Source: CAD feature listing. Evaluate the final solid. Frame: model axes, mm. Face numbers are marked on the shaded views. Give positions to 0.01 mm unless a question says otherwise; leave off trailing zeros. Order: outer loops, then holes, each group sorted by start corner. A loop starts at its lowest first (then second) coordinate and runs counter-clockwise, first axis right, second up.
from build123d import *

# Parameters (mm, degrees)
SALIENTE_EXTRUIR1_DEPTH = 75
SALIENTE_EXTRUIR2_START = -17
SALIENTE_EXTRUIR2_DEPTH = 17.566243
CROQUIS3_R              = 3.96875
CORTAR_EXTRUIR1_DEPTH   = 10
CROQUIS4_R              = 6.46875
CROQUIS4_R_2            = 3.96875
CORTAR_EXTRUIR2_DEPTH   = 3
SALIENTE_EXTRUIR3_START = -6.919182
CROQUIS7_R              = 1.984375
SALIENTE_EXTRUIR3_DEPTH = 6.919182
CORTAR_EXTRUIR3_DEPTH   = 75
CROQUIS9_R              = 1
CORTAR_EXTRUIR4_DEPTH   = 10


with BuildPart() as part:
    # Croquis1 → Saliente-Extruir1 (new body, symmetric)
    with BuildSketch(Plane.XY):
        with BuildLine():
            ThreePointArc((-1.339746, 5), (14.365661, 8.57646), (28, 0))
            Line((28, 0), (28, -10))
            Line((28, -10), (25, -10))
            Line((25, -10), (25, 0))
            Line((25, 0), (0, 0))
            Line((0, 0), (-60.621778, -35))
            Line((-60.621778, -35), (-70.621778, -35))
            Line((-70.621778, -35), (-1.339746, 5))
        make_face()
    extrude(amount=SALIENTE_EXTRUIR1_DEPTH, both=True)

    # Croquis2 → Saliente-Extruir2 (add)
    with BuildSketch(Plane(origin=(0, -15, 0), x_dir=(1, 0, 0), z_dir=(0, 1, 0)).offset(SALIENTE_EXTRUIR2_START)):
        with BuildLine():
            Line((-32.5, 4.330127), (-32.5, 12.5))
            Line((-32.5, 12.5), (-27.5, 12.5))
            Line((-27.5, 12.5), (-27.5, 4.330127))
            ThreePointArc((-27.5, 4.330127), (-25, 0), (-27.5, -4.330127))
            Line((-27.5, -4.330127), (-27.5, -12.5))
            Line((-27.5, -12.5), (-32.5, -12.5))
            Line((-32.5, -12.5), (-32.5, -4.330127))
            ThreePointArc((-32.5, -4.330127), (-35, 0), (-32.5, 4.330127))
        make_face()
        with BuildLine():
            Line((-32.5, 54.330127), (-32.5, 62.5))
            Line((-32.5, 62.5), (-27.5, 62.5))
            Line((-27.5, 62.5), (-27.5, 54.330127))
            ThreePointArc((-27.5, 54.330127), (-25, 50), (-27.5, 45.669873))
            Line((-27.5, 45.669873), (-27.5, 37.5))
            Line((-27.5, 37.5), (-32.5, 37.5))
            Line((-32.5, 37.5), (-32.5, 45.669873))
            ThreePointArc((-32.5, 45.669873), (-35, 50), (-32.5, 54.330127))
        make_face()
        with BuildLine():
            Line((-32.5, -45.669873), (-32.5, -37.5))
            Line((-32.5, -37.5), (-27.5, -37.5))
            Line((-27.5, -37.5), (-27.5, -45.669873))
            ThreePointArc((-27.5, -45.669873), (-25, -50), (-27.5, -54.330127))
            Line((-27.5, -54.330127), (-27.5, -62.5))
            Line((-27.5, -62.5), (-32.5, -62.5))
            Line((-32.5, -62.5), (-32.5, -54.330127))
            ThreePointArc((-32.5, -54.330127), (-35, -50), (-32.5, -45.669873))
        make_face()
    extrude(amount=SALIENTE_EXTRUIR2_DEPTH)

    # Croquis3 → Cortar-Extruir1 (cut)
    with BuildSketch(Plane(origin=(0, 8.875562, 0), x_dir=(1, 0, 0), z_dir=(0, 1, 0))):
        with Locations((14, -50)):
            Circle(CROQUIS3_R)
        with Locations((14, 0)):
            Circle(CROQUIS3_R)
        with Locations((14, 50)):
            Circle(CROQUIS3_R)
    extrude(amount=-CORTAR_EXTRUIR1_DEPTH, mode=Mode.SUBTRACT)

    # Croquis4 → Cortar-Extruir2 (cut)
    with BuildSketch(Plane(origin=(0, 8.875562, 0), x_dir=(1, 0, 0), z_dir=(0, 1, 0))):
        with Locations((14, 50)):
            Circle(CROQUIS4_R)
        with Locations((14, 50)):
            Circle(CROQUIS4_R_2, mode=Mode.SUBTRACT)
        with Locations((14, 0)):
            Circle(CROQUIS4_R)
        with Locations((14, 0)):
            Circle(CROQUIS4_R_2, mode=Mode.SUBTRACT)
        with Locations((14, -50)):
            Circle(CROQUIS4_R)
        with Locations((14, -50)):
            Circle(CROQUIS4_R_2, mode=Mode.SUBTRACT)
    extrude(amount=-CORTAR_EXTRUIR2_DEPTH, mode=Mode.SUBTRACT)

    # Croquis7 → Saliente-Extruir3 (add)
    with BuildSketch(Plane(origin=(0, -35, 0), x_dir=(-1, 0, 0), z_dir=(0, -1, 0)).offset(SALIENTE_EXTRUIR3_START)):
        with Locations((50.621778, 0)):
            Circle(CROQUIS7_R)
        with Locations((50.621778, 50)):
            Circle(CROQUIS7_R)
        with Locations((50.621778, -50)):
            Circle(CROQUIS7_R)
    extrude(amount=SALIENTE_EXTRUIR3_DEPTH)

    # Croquis8 → Cortar-Extruir3 (cut, symmetric)
    with BuildSketch(Plane.XY):
        with BuildLine():
            ThreePointArc((-50.621778, -35), (-51.865537, -34.582808), (-52.606153, -33.5))
            Line((-52.606153, -33.5), (-52.606153, -35))
            Line((-52.606153, -35), (-50.621778, -35))
        make_face()
        with BuildLine():
            ThreePointArc((-48.637403, -33.5), (-49.378019, -34.582808), (-50.621778, -35))
            Line((-50.621778, -35), (-48.637403, -35))
            Line((-48.637403, -35), (-48.637403, -33.5))
        make_face()
    extrude(amount=CORTAR_EXTRUIR3_DEPTH, both=True, mode=Mode.SUBTRACT)

    # Croquis9 → Cortar-Extruir4 (cut)
    with BuildSketch(Plane.XZ.offset(32)):
        with Locations((-30, 0)):
            Circle(CROQUIS9_R)
        with Locations((-30, 50)):
            Circle(CROQUIS9_R)
        with Locations((-30, -50)):
            Circle(CROQUIS9_R)
    extrude(amount=-CORTAR_EXTRUIR4_DEPTH, mode=Mode.SUBTRACT)


solid = part.part
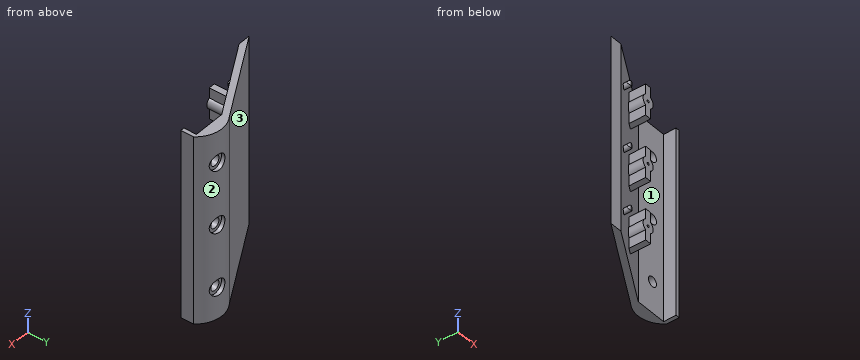
1) Section query D-D on z = -22. Output: boundary loops of the cut face in (x, y).
Checks:
outline: (-70.62, -35) - (-60.62, -35) - (0, 0) - (25, 0) - (25, -10) - (28, -10) - (28, 0) arc R21.05 ccw to (-1.34, 5) - close
2) Section query C-C on x = 14. Output: boundary loops of the cut face in (y, z).
Checks:
outline: (0, -75) - (8.64, -75) - (8.64, -56.47) - (5.88, -56.47) - (5.88, -53.97) - (0, -53.97) - close; (0, -46.03) - (5.88, -46.03) - (5.88, -43.53) - (8.64, -43.53) - (8.64, -6.47) - (5.88, -6.47) - (5.88, -3.97) - (0, -3.97) - close; (0, 3.97) - (5.88, 3.97) - (5.88, 6.47) - (8.64, 6.47) - (8.64, 43.53) - (5.88, 43.53) - (5.88, 46.03) - (0, 46.03) - close; (0, 53.97) - (5.88, 53.97) - (5.88, 56.47) - (8.64, 56.47) - (8.64, 75) - (0, 75) - close
3) Ray query, L1, parallel to Z at x = -30, y = -25; L2, parallel to Z at x = 14, y = 3.3; L3, parallel to Z at x = 14, y = 6. Return the intervals inside material, ascending.
Checks:
L1: z = -62.5 to -51, -49 to -37.5, -12.5 to -1, 1 to 12.5, 37.5 to 49, 51 to 62.5
L2: z = -75 to -53.97, -46.03 to -3.97, 3.97 to 46.03, 53.97 to 75
L3: z = -75 to -56.47, -43.53 to -6.47, 6.47 to 43.53, 56.47 to 75
4) First-contact query: pin 1 Ø10.5 at (x, z) = (14, -50) entering from -Y; pin 2 Ø3 at (y, z) = (-2.5, -6) entering from -X; pin 3 Ø1.5 at (x, y) = (-31, -21.5) entering from +Z; pin 4 Ø3 at (x, y) = (-29.5, -8) entering from -Z. Flat tips, straight axial feed; report the tip coordinate or a pass-through.
Checks:
pin 1: stops at y = 0
pin 2: stops at x = -16.93
pin 3: stops at z = 62.5
pin 4: passes through
5) Pull-direction query (X, two-part tool) for the marked faces 1, 2 and 3; classes: +X half, -X half, draft (parallel to the pull), parting line (faces both ways), or undercut.
Checks:
face 1: undercut
face 2: parting line
face 3: -X half
6) Section query B-B on z = -61. Output: boundary loops of the cut face in (x, y).
Checks:
outline: (-70.62, -35) - (-60.62, -35) - (-32.5, -18.76) - (-32.5, -32) - (-27.5, -32) - (-27.5, -15.88) - (0, 0) - (25, 0) - (25, -10) - (28, -10) - (28, 0) arc R21.05 ccw to (-1.34, 5) - close
7) Section query A-A on y = -2. Output: boundary loops of the cut face in (x, z).
Checks:
outline: (-13.46, -75) - (-3.46, -75) - (-3.46, 75) - (-13.46, 75) - close; (25, -75) - (28, -75) - (28, 75) - (25, 75) - close
